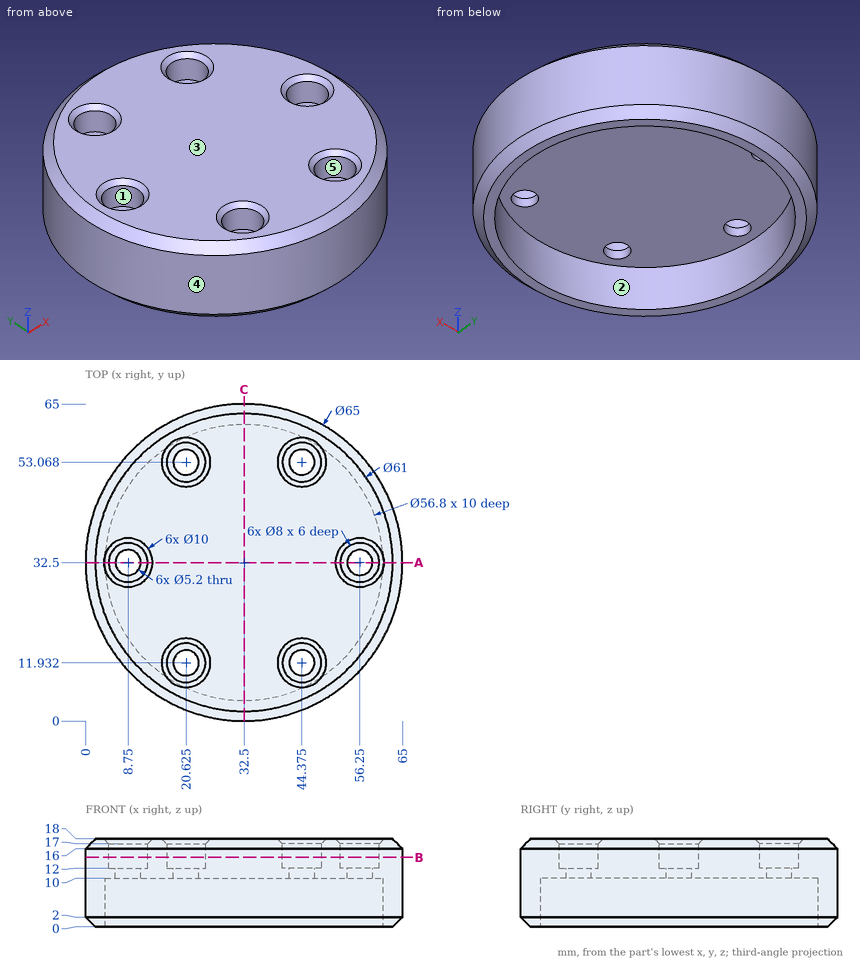
Drawing for the job (mm, zero at the part's lowest x, y, z). A direction names the side the tool comes from. Round coordinates to 2 decimals unless told otherwise and drop trailing zeros. Loops run counter-clockwise (first coordinate to the right, second up) from the corner with the lowest first, then second, coordinate; pieces in that order, holes last. Notation, with made-up numbers: (77.5, 65) -> (111.5, 65) arc R26 cw to (111.5, 82) -> close; hole circle Ø6 at (55.5, -11.5). An arc over 180 degrees is marked (long way). Use one line per item in the form item = value. Start each with the question number.
Item 1: Band-saw the part on A-A (y = 32.5). Give the number of separate pieces and of enclosed holes in the cut face, plus the area to 3 significant figures.
Item 2: Two-plate mould, pull along Y, no slides. Class the marked faces 3, 4 and 5: released by +Y, released by -Y, zero draft, split by the parting line, or undercut.
Item 3: Drop flat-ended pins along their axis: pin 1 Ø7 at (x, y) = (20.62, 11.93) entering from -Z; pin 2 Ø6.5 at (x, y) = (44, 10.5) entering from +Z; pin 3 Ø5 at (x, z) = (33.5, 4.5) entering from +Y; pin 4 Ø4 at (x, y) = (56.25, 32.5) entering from -Z. Give the stop position or say it passes through.
Item 4: Band-saw the part on B-B (z = 14.25). List the corners of the cut face in (x, y) (3 decimals), plus the area to 3 significant figures.
Item 5: Drill centre lines: line 1 along X through (y, z) = (13.5, 16) (1 decimal); line 2 along Y through (x, z) = (32, 2) (1 decimal); line 3 along Y through (x, z) = (19.5, 6.25). Where is each one in solid material? Low to high.
Item 6: Band-saw the part on C-C (x = 32.5). List the corners of the cut face in (y, z), plus the area to 3 significant figures.
Item 7: Tool access for the marked faces 1 and 2: list every direction of +Z, -Z, +X, -X, +Y, -Y with a clear straight run to the whole face (end or side of a thin tool).
Data:
q1.separate_pieces = 3
q1.enclosed_holes = 0
q1.area = 475 mm^2
q2.face_3 = zero draft
q2.face_4 = split by the parting line
q2.face_5 = undercut
q3.pin_1 = 10
q3.pin_2 = 17.73
q3.pin_3 = 65
q3.pin_4 = through
q4.outline = circle Ø65 at (32.5, 32.5); hole circle Ø8 at (8.75, 32.5); hole circle Ø8 at (20.625, 11.932); hole circle Ø8 at (20.625, 53.068); hole circle Ø8 at (44.375, 11.932); hole circle Ø8 at (44.375, 53.068); hole circle Ø8 at (56.25, 32.5)
q4.area = 3,020 mm^2
q5.line_1 = 6.1 to 16.9, 24.3 to 40.7, 48.1 to 58.9
q5.line_2 = 0 to 4.1, 60.9 to 65
q5.line_3 = 2.71 to 7.25, 57.75 to 62.29
q6.outline = (0, 2) -> (2, 0) -> (4.1, 0) -> (4.1, 10) -> (60.9, 10) -> (60.9, 0) -> (63, 0) -> (65, 2) -> (65, 16) -> (63, 18) -> (2, 18) -> (0, 16) -> close
q6.area = 594 mm^2
q7.face_1 = +Z
q7.face_2 = -Z
